```python
from build123d import *

# Parameters (mm, degrees)
ESBO_O1_W                = 19
ESBO_O1_H                = 3
RESSALTO_EXTRUS_O1_DEPTH = 2


with BuildPart() as part:
    # Esboço1 → Ressalto-extrusão1 (new body)
    with BuildSketch(Plane(origin=(0, 0, 0), x_dir=(1, 0, 0), z_dir=(0, 1, 0))):
        Polygon((-10.479474548, 11.375), (12.520525452, 11.375), (12.520525452, -0.625), (10.520525452, -0.625), (-10.479474548, -0.625), (-10.479474548, 6.375), (10.520525452, 6.375), (10.520525452, 9.375), (-10.479474548, 9.375), align=None)
        with Locations((1.020525452, 2.875)):
            Rectangle(ESBO_O1_W, ESBO_O1_H, mode=Mode.SUBTRACT)
    extrude(amount=RESSALTO_EXTRUS_O1_DEPTH)


solid = part.part
```
Geometry check sheet. Reference: the model listing, model coordinates, mm. A direction names the side the tool comes from. Coordinates: 2 decimals unless noted, no trailing zeros. Order: outer loops, then holes, each group sorted by start corner. A loop starts at its lowest first (then second) coordinate and runs counter-clockwise, first axis right, second up.
Item 1: Section check B-B (y = 1.1). Enter the section's corners in (x, z) (3 decimals), plus the area to 3 significant figures.
Item 2: Mould release check, pull along X, two halves, no side actions. Record for faces 4 (the flat face through (1, 0, -5)), 5 (the flat face through (12.521, 1, -5)), 6 (the flat face through (1, 1, -1.375)): released by +X, released by -X, zero draft, split by the parting line, or undercut.
Item 3: Section check C-C (z = -8.5). Enter the section's corners in (x, y), plus the area to 3 significant figures.
Item 4: Depth check by flat-ended pin: pin 1 (6 mm diameter, centred on x = 8.5, z = -2.5, fed in from -Y). Enter the tip coordinate at first touch or a pass-through.
Item 5: Tool access check on faces 1 (the flat face through (10.521, 1, -3)), 2 (the flat face through (10.521, 1, -8)), 3 (the flat face through (1, 1, -11.375)). Record the directions out of +Z, -Z, +X, -X, +Y, -Y that give a thin tool (end or side, any length) a straight path to the whole face; none if there is none.
Item 6: Section check A-A (x = 3). Enter the section's corners in (y, z) (3 decimals), plus the area to 3 significant figures.
Item 7: Scan lines: line 1 along Z through (x, y) = (-5, 1.2) (3 decimals); line 2 along X through (y, z) = (0.55, -3.75); line 3 along X through (y, z) = (1.9, -9.25). Record each from-to range of solid material in increasing order.
Check sheet entries:
1. outline: (-10.479, -11.375) - (12.521, -11.375) - (12.521, 0.625) - (-10.479, 0.625) - (-10.479, -6.375) - (10.521, -6.375) - (10.521, -9.375) - (-10.479, -9.375) - close; hole (-8.479, -4.375) - (10.521, -4.375) - (10.521, -1.375) - (-8.479, -1.375) - close
1. area: 156 mm2
2. face 4: zero draft
2. face 5: released by +X
2. face 6: undercut
3. outline: (10.52, 0) - (12.52, 0) - (12.52, 2) - (10.52, 2) - close
3. area: 4.00 mm2
4. pin 1: stops at y = 0
5. face 1: +Y, -Y
5. face 2: -X, +Y, -Y
5. face 3: -Z, +X, -X, +Y, -Y
6. outline: (0, -11.375) - (2, -11.375) - (2, -9.375) - (0, -9.375) - close; (0, -6.375) - (2, -6.375) - (2, -4.375) - (0, -4.375) - close; (0, -1.375) - (2, -1.375) - (2, 0.625) - (0, 0.625) - close
6. area: 12.0 mm2
7. line 1: z = -11.375 to -9.375, -6.375 to -4.375, -1.375 to 0.625
7. line 2: x = -10.48 to -8.48, 10.52 to 12.52
7. line 3: x = 10.52 to 12.52
